For this review, use the dimensioned drawing (mm, ordinates from the lowest corner) and the shaded views. A direction names the side the tool comes from. Round coordinates to 2 decimals unless told otherwise and drop trailing zeros. Order: outer loops, then holes, each group sorted by start corner. A loop starts at its lowest first (then second) coordinate and runs counter-clockwise, first axis right, second up. Notation, with made-up numbers: (33.25, -31) - (43.25, -31) arc R11 cw to (43.25, -23) - close; hole circle Ø10 at (4, -0.5). An arc over 180 degrees is marked (long way). Use CSV: the item, a comma, the result in double quotes. Start each with the question number.
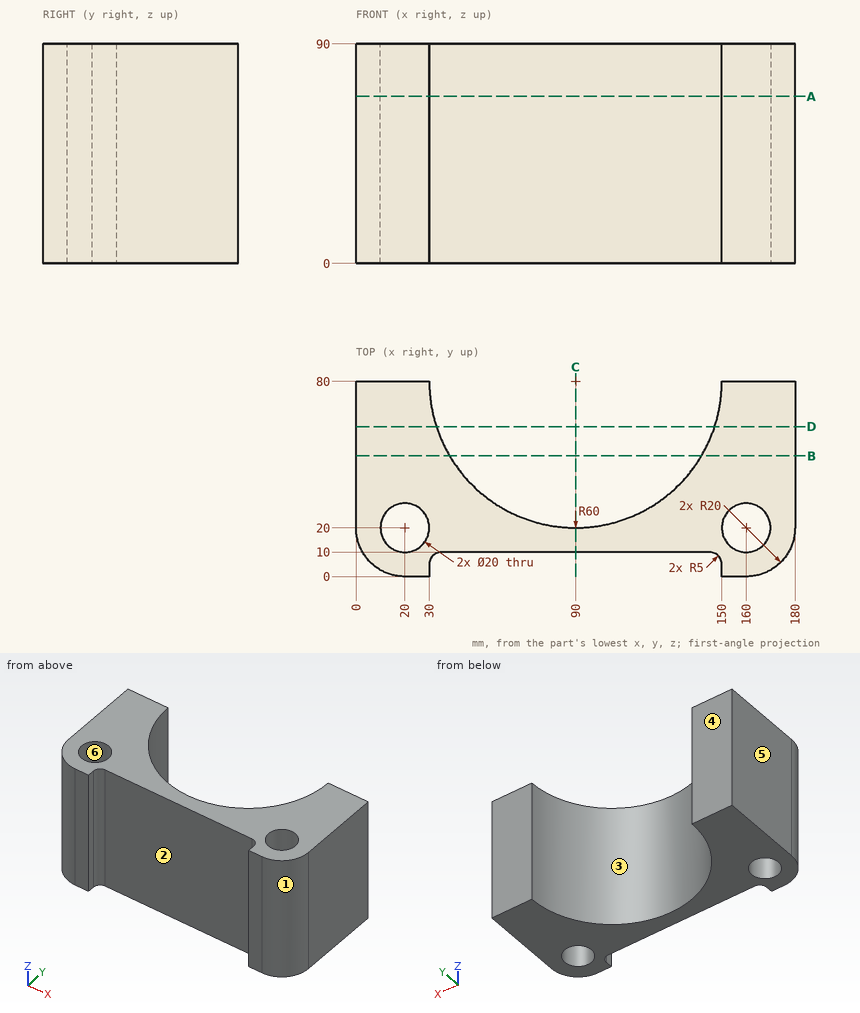
Q1. Take a section at A-A (z = 68.5). State the section outline as (x, y) points, plus the area to 3 significant figures.
Q2. The part is to be moulded in two halves that separate along X. For the marked faces 3, 4, 5 and 6, say which applies: +X half, -X half, draft (parallel to the pull), parting line (faces both ways), or undercut.
Q3. For L1, parallel to Y at x = 20, z = 50; L2, parallel to X at y = 16, z = 24.5; L3, parallel to X at y = 28, z = 73, list the stretches that pass through material, from the lowest coordinate up. Write a range as [from, to].
Q4. Take a section at D-D (y = 61.5). State the section outline as (x, z) points, plus the area to 3 significant figures.
Q5. Take a section at B-B (y = 49.5). State the section outline as (x, z) points.
Q6. Tool access review of the marked faces 1 and 2: name each direction out of +Z, -Z, +X, -X, +Y, -Y from which nothing blocks a thin tool from reaching the whole face with its end or side.
Q7. Clearance check with flat-ended pins moving along their axes: pin 1 (1.5 mm diameter, centred on y = 1.5, z = 67, fed in from +X); pin 2 (1.5 mm diameter, centred on y = 1.5, z = 65.5, fed in from -X); pin 3 (2 mm diameter, centred on x = 92.5, z = 44.5, fed in from +Y); pin 4 (8 mm diameter, centred on x = 21, z = 32, fed in from -Y). State where each tip first meets the part, or that it passes through.
Q8. Take a section at C-C (x = 90). State the section outline as (y, z) points, plus the area to 3 significant figures.
Findings below:
1,outline,"(0, 20) arc R20 ccw to (20, 0) - (30, 0) - (30, 5) arc R5 cw to (35, 10) - (145, 10) arc R5 cw to (150, 5) - (150, 0) - (160, 0) arc R20 ccw to (180, 20) - (180, 80) - (150, 80) arc R60 cw to (30, 80) - (0, 80) - close; hole circle Ø20 at (20, 20); hole circle Ø20 at (160, 20)"
1,area,"6,760 mm^2"
2,face 3,"undercut"
2,face 4,"draft"
2,face 5,"-X half"
2,face 6,"undercut"
3,L1,"y = [0, 10], [30, 80]"
3,L2,"x = [0.4, 10.83], [29.17, 150.83], [169.17, 179.6]"
3,L3,"x = [0, 14], [26, 60.07], [119.93, 154], [166, 180]"
4,outline,"(0, 0) - (32.92, 0) - (32.92, 90) - (0, 90) - close; (147.08, 0) - (180, 0) - (180, 90) - (147.08, 90) - close"
4,area,"5,930 mm^2"
5,outline,"(0, 0) - (38.33, 0) - (38.33, 90) - (0, 90) - close; (141.67, 0) - (180, 0) - (180, 90) - (141.67, 90) - close"
6,face 1,"+Z, -Z, +X, -Y"
6,face 2,"+Z, -Z, -Y"
7,pin 1,"stops at x = 169.22"
7,pin 2,"stops at x = 10.78"
7,pin 3,"stops at y = 20.1"
7,pin 4,"stops at y = 0"
8,outline,"(10, 0) - (20, 0) - (20, 90) - (10, 90) - close"
8,area,"900 mm^2"
